```python
from build123d import *

# Parameters (mm, degrees)
SKETCH1_W           = 30
SKETCH1_H           = 10
BOSS_EXTRUDE1_DEPTH = 2
SKETCH2_R           = 2.5
BOSS_EXTRUDE2_DEPTH = 10
LPATTERN1_COUNT     = 2
LPATTERN1_PITCH     = 20
SKETCH3_R           = 2.5
CUT_EXTRUDE1_DEPTH  = 10


with BuildPart() as part:
    # Sketch1 → Boss-Extrude1 (new body)
    with BuildSketch(Plane.XY):
        Rectangle(SKETCH1_W, SKETCH1_H)
    extrude(amount=BOSS_EXTRUDE1_DEPTH)

    # Sketch2 → Boss-Extrude2 (add)
    with BuildSketch(Plane.ZY.offset(15)):
        with BuildLine():
            Line((0, 5), (0, 10))
            ThreePointArc((0, 10), (6.458039892, 11.870828693), (2, 6.83772234))
            Line((2, 6.83772234), (2, 5))
            Line((2, 5), (0, 5))
        make_face()
        with Locations((3.5, 10)):
            Circle(SKETCH2_R, mode=Mode.SUBTRACT)
    boss_extrude2 = extrude(amount=-BOSS_EXTRUDE2_DEPTH)

    # LPattern1: Boss-Extrude2 ×2
    with Locations(*[(i * LPATTERN1_PITCH, 0, 0) for i in range(1, LPATTERN1_COUNT)]):
        add(boss_extrude2)

    # Sketch3 → Cut-Extrude1 (cut)
    with BuildSketch(Plane.XY.offset(2)):
        with Locations((-10, 0)):
            Circle(SKETCH3_R)
        Circle(SKETCH3_R)
        with Locations((10, 0)):
            Circle(SKETCH3_R)
    extrude(amount=-CUT_EXTRUDE1_DEPTH, mode=Mode.SUBTRACT)


solid = part.part
```
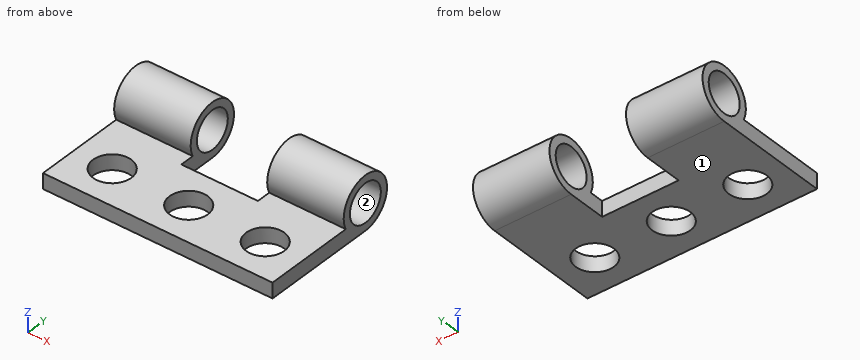
Work out the finished part from the listing and answer in its coordinate system (mm). Face numbers are marked on the shaded views. Round coordinates to 2 decimals unless told otherwise and drop trailing zeros. Write each loop counter-clockwise with the first axis right and the second up, starting at its lowest first coordinate (ties: lowest second). Pieces come first, ordered by that corner, then holes. Notation, with made-up numbers: (14.5, 18.25) -> (42.5, 18.25) arc R30 cw to (42.5, 53.25) -> close; hole circle Ø3 at (14.25, 4.5). An arc over 180 degrees is marked (long way). Write each question's results on one line, items separated by ' | '.
1) The part is cut by section B-B (x = 0). Write down the section's boundary in (y, z).
Findings:
outline: (-5, 0) -> (-2.5, 0) -> (-2.5, 2) -> (-5, 2) -> close; (2.5, 0) -> (5, 0) -> (5, 2) -> (2.5, 2) -> close
2) Consider line 1 along Y through (x, z) = (11.5, 3.5); line 2 along Y through (x, z) = (0, 0.5); line 3 along X through (y, z) = (6.75, 1.5). Determine where each line is inside the solid, lowest interval first. Write a range as [from, to].
Findings:
line 1: y = [6.5, 7.5], [12.5, 13.5] | line 2: y = [-5, -2.5], [2.5, 5] | line 3: x = [-15, -5], [5, 15]
3) The part is cut by section C-C (y = 0). Write down the section's boundary in (x, z), and give its area (3 significant figures).
Findings:
outline: (-15, 0) -> (-12.5, 0) -> (-12.5, 2) -> (-15, 2) -> close; (-7.5, 0) -> (-2.5, 0) -> (-2.5, 2) -> (-7.5, 2) -> close; (2.5, 0) -> (7.5, 0) -> (7.5, 2) -> (2.5, 2) -> close; (12.5, 0) -> (15, 0) -> (15, 2) -> (12.5, 2) -> close | area: 30.0 mm²
4) The part is cut by section A-A (x = -10). Write down the section's boundary in (y, z).
Findings:
outline: (-5, 0) -> (-2.5, 0) -> (-2.5, 2) -> (-5, 2) -> close; (2.5, 0) -> (10, 0) arc R3.5 ccw (long way) to (6.84, 2) -> (2.5, 2) -> close; hole circle Ø5 at (10, 3.5)
5) Flat-ended cylindrical pins translate along their axes: pin 1 (4 mm diameter, centred on y = 10, z = 3.5, fed in from +X); pin 2 (2 mm diameter, centred on x = 2.5, z = 1.5, fed in from +Y); pin 3 (1 mm diameter, centred on y = 6.5, z = 2.5, fed in from +X). Find the tip coordinate at first contact, or state that the pin passes through.
Findings:
pin 1: passes through | pin 2: stops at y = 5 | pin 3: stops at x = 15
6) For a pull along Z with two mould halves and no side action, classify the marked faces 1 and 2 as +Z half, -Z half, draft (parallel to the pull), parting line (faces both ways), or undercut.
Findings:
face 1: -Z half | face 2: undercut
7) The part is cut by section D-D (z = 3.5). Write down the section's boundary in (x, y).
Findings:
outline: (-15, 6.5) -> (-5, 6.5) -> (-5, 7.5) -> (-15, 7.5) -> close; (-15, 12.5) -> (-5, 12.5) -> (-5, 13.5) -> (-15, 13.5) -> close; (5, 6.5) -> (15, 6.5) -> (15, 7.5) -> (5, 7.5) -> close; (5, 12.5) -> (15, 12.5) -> (15, 13.5) -> (5, 13.5) -> close
